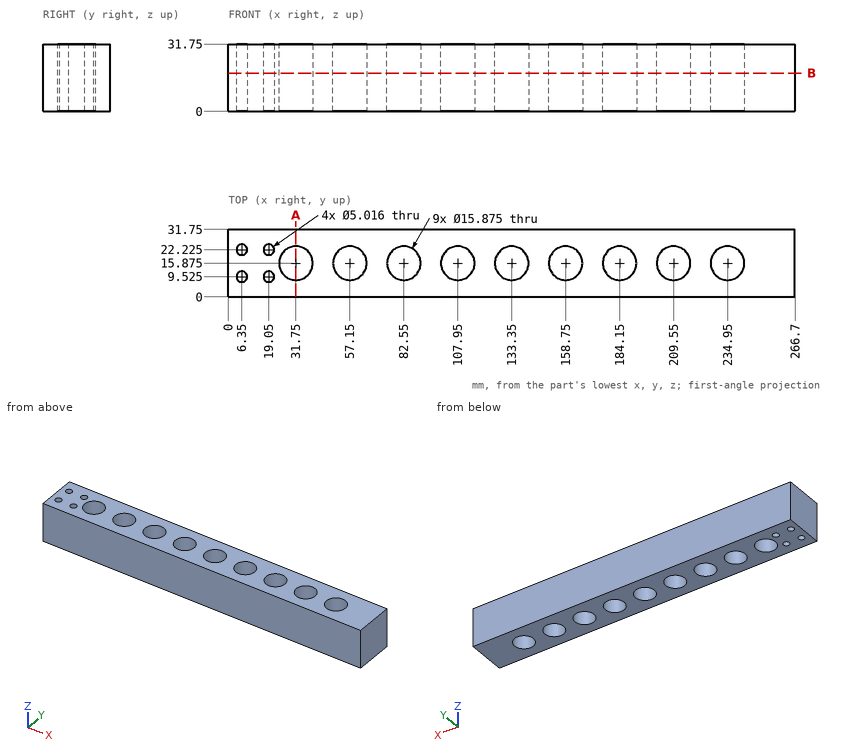
Source: three-view drawing plus pictorial views. Frame: mm from the lowest corner of the part. Give positions to 0.01 mm unless a question says otherwise; leave off trailing zeros. Write each loop counter-clockwise with the first axis right and the second up, starting at its lowest first coordinate (ties: lowest second). Pieces come first, ordered by that corner, then holes.
(1) Cut plane A-A, the plane x = 31.75. Return loops of the section in (y, z).
(2) Cut plane B-B, the plane z = 18. Give the number of separate pieces and of enclosed holes in the cut face, then the cut area to 3 significant figures.
(3) Ray query, line 1 (Y direction, x = 6, z = 20); line 2 (Y direction, x = 158, z = 11); line 3 (Y direction, x = 57.15, z = 19). Return the intervals inside material, ascending.
Values follow:
1. outline: (0, 0) - (7.94, 0) - (7.94, 31.75) - (0, 31.75) - close; (23.81, 0) - (31.75, 0) - (31.75, 31.75) - (23.81, 31.75) - close
2. separate pieces: 1
2. enclosed holes: 13
2. area: 6,610 mm2
3. line 1: y = 0 to 7.04, 12.01 to 19.74, 24.71 to 31.75
3. line 2: y = 0 to 7.97, 23.78 to 31.75
3. line 3: y = 0 to 7.94, 23.81 to 31.75
